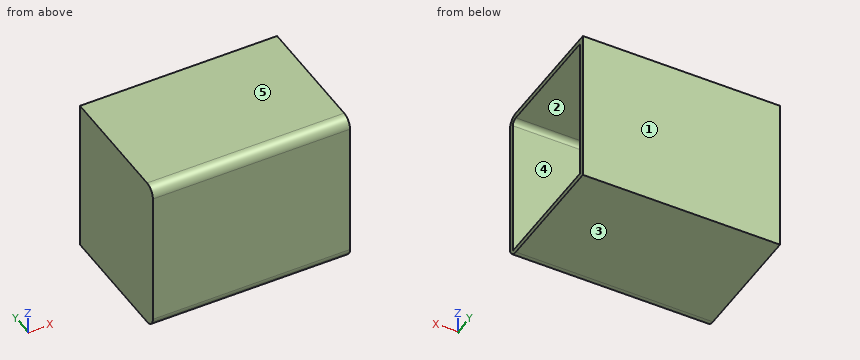
```python
from build123d import *

# Parameters (mm, degrees)
F0_W     = 95.25
F0_H     = 63.5
F1_DEPTH = 76.2
F2_R     = 5.08
F3_T     = -2.54
F4_R     = 5.08


with BuildPart() as f1:
    # F0 (on Top) → F1 (new body)
    with BuildSketch(Plane.XY):
        with Locations((47.625, 31.75)):
            Rectangle(F0_W, F0_H)
    extrude(amount=F1_DEPTH)

    # F2
    f2_edges = [f1.edges().sort_by_distance(p)[0] for p in [
        (47.625, 0, 76.2),
    ]]
    fillet(f2_edges, radius=F2_R)

    # F3
    f3_openings = [f1.faces().sort_by_distance(p)[0] for p in [
        (95.25, 31.785081, 38.057643),
    ]]
    offset(amount=F3_T, openings=f3_openings)

    # F4
    f4_edges = [f1.edges().sort_by_distance(p)[0] for p in [
        (47.625, 0, 0),
    ]]
    fillet(f4_edges, radius=F4_R)


solid = f1.part
```
The model under review builds one solid part; all positions refer to its coordinate system, in mm. Face numbers are marked on the shaded views. A direction names the side the tool comes from. Give positions to 0.01 mm unless a question says otherwise; leave off trailing zeros. Write each loop counter-clockwise with the first axis right and the second up, starting at its lowest first coordinate (ties: lowest second). Pieces come first, ordered by that corner, then holes. Notation, with made-up numbers: (10, -27) -> (14, -27) arc R20 cw to (14, -13) -> close; hole circle Ø1 at (-22, 83). An arc over 180 degrees is marked (long way). Answer in a Markdown table with one row per item.
1) For L1, parallel to Z at x = 25.5, y = 26.5; L2, parallel to Y at x = 86.5, z = 50; L3, parallel to X at y = 57.5, z = 43, list the stretches that pass through material, from the lowest coordinate up. Write a range as [from, to].
Worked answers:
| item | result |
|---|---|
| L1 | [0, 2.54], [73.66, 76.2] |
| L2 | [0, 2.54], [60.96, 63.5] |
| L3 | [0, 2.54] |
2) Mouldability with a two-part tool opening along Y and no side actions: class the marked faces 1, 2 and 3 as +Y half, -Y half, draft (parallel to the pull), parting line (faces both ways), or undercut.
Worked answers:
| item | result |
|---|---|
| face 1 | +Y half |
| face 2 | undercut |
| face 3 | draft |
3) Clearance check with a flat-ended pin moving along its axis: P1, Ø1.5, axis at y = 56.5, z = 18.5, coming from the +X side. State where the tip first meets the part, or that it passes through.
Worked answers:
| item | result |
|---|---|
| P1 | x = 2.54 |
4) Add section B-B on z = 13. State the section outline as (x, y) points.
Worked answers:
| item | result |
|---|---|
| outline | (0, 0) -> (95.25, 0) -> (95.25, 2.54) -> (2.54, 2.54) -> (2.54, 60.96) -> (95.25, 60.96) -> (95.25, 63.5) -> (0, 63.5) -> close |
5) Add section A-A on x = 50. State the section outline as (y, z) points.
Worked answers:
| item | result |
|---|---|
| outline | (0, 5.08) arc R5.08 ccw to (5.08, 0) -> (63.5, 0) -> (63.5, 76.2) -> (5.08, 76.2) arc R5.08 ccw to (0, 71.12) -> close; hole (2.54, 2.54) -> (60.96, 2.54) -> (60.96, 73.66) -> (5.08, 73.66) arc R2.54 ccw to (2.54, 71.12) -> close |
6) Tool access review of the marked faces 4 and 5: name each direction out of +Z, -Z, +X, -X, +Y, -Y from which nothing blocks a thin tool from reaching the whole face with its end or side.
Worked answers:
| item | result |
|---|---|
| face 4 | +X |
| face 5 | +Z, +X, -X, +Y, -Y |
7) Add section C-C on y = 14.5. State the section outline as (x, z) points.
Worked answers:
| item | result |
|---|---|
| outline | (0, 0) -> (95.25, 0) -> (95.25, 2.54) -> (2.54, 2.54) -> (2.54, 73.66) -> (95.25, 73.66) -> (95.25, 76.2) -> (0, 76.2) -> close |
